from build123d import *

# Parameters (mm, degrees)
BOSS_EXTRUDE1_START = -203.2
BOSS_EXTRUDE1_DEPTH = 203.2
SKETCH15_R          = 5
CUT_EXTRUDE1_DEPTH  = 15


with BuildPart() as part:
    # Sketch12 → Revolve1 (revolve)
    with BuildSketch(Plane.XY, mode=Mode.PRIVATE) as revolve1_sk:
        Polygon((-25.399999994, 0), (-25.399999994, 203.2), (-20.955, 203.2), (-20.955, 165.1), (-19.177, 165.1), (-19.177, 38.1), (-20.955, 38.1), (-20.955, 0), align=None)
    revolve(revolve1_sk.sketch.rotate(Axis((0, 0, 0), (0, 1, 0)), 270), axis=Axis((0, 0, 0), (0, 1, 0)))

    # Sketch13 → Boss-Extrude1 (add)
    with BuildSketch(Plane(origin=(0, 0, 0), x_dir=(-1, 0, 0), z_dir=(0, -1, 0)).offset(BOSS_EXTRUDE1_START)):
        with BuildLine():
            Line((12.584838028, 40.399999994), (-25.399999994, 40.399999994))
            Line((-25.399999994, 40.399999994), (-25.399999994, 0))
            ThreePointArc((-25.399999994, 0), (0, 25.399999994), (25.399999994, 0))
            Line((25.399999994, 0), (25.399999994, 40.399999994))
            Line((25.399999994, 40.399999994), (22.584838028, 40.399999994))
            Line((22.584838028, 40.399999994), (12.584838028, 40.399999994))
        make_face()
    extrude(amount=BOSS_EXTRUDE1_DEPTH)

    # Sketch15 → Cut-Extrude1 (cut)
    with BuildSketch(Plane(origin=(0, 0, -40.399999994), x_dir=(-1, 0, 0), z_dir=(0, 0, -1))):
        with Locations((-12.699999997, 30)):
            Circle(SKETCH15_R)
        with Locations((-12.699999997, 173.2)):
            Circle(SKETCH15_R)
    cut_extrude1 = extrude(amount=-CUT_EXTRUDE1_DEPTH, mode=Mode.SUBTRACT)

    # Mirror1: Cut-Extrude1 across plane
    add(cut_extrude1.mirror(Plane(origin=(0, 0, 0), x_dir=(0, 0, 1), z_dir=(1, 0, 0))), mode=Mode.SUBTRACT)


solid = part.part
Can you work these out from the model? Positions are in its coordinate system, mm. A direction names the side the tool comes from. Coordinates: 2 decimals unless noted, no trailing zeros. Loops run counter-clockwise (first coordinate to the right, second up) from the corner with the lowest first, then second, coordinate; pieces in that order, holes last. Notation, with made-up numbers: (-3, 72.25) - (6, 72.25) arc R29 cw to (6, 103.25) - close; hole circle Ø2 at (-25.5, 46.5). An arc over 180 degrees is marked (long way). Put each result on its own line as item: value. Start each with the question number.
Item 1: Which directions (+Z, -Z, +X, -X, +Y, -Y) give clear straight access to the entire face, cutting with the end or side of a thin tool? Please do faces 1 (the face through (-13, 173, -25.4)), 2 (the face through (0, 203.2, -23)), 3 (the face through (17, 38.1, 9.2)), 4 (the face through (0, 103, -40.4)), 5 (the face through (-17.669, 183.883, -11.265)).
Item 2: If we mould it in two halves opening along Z, with no side actions, what happens to faces 6 (the face through (-17.669, 18.783, -11.265)), 7 (the face through (-19.014, 100.711, 2.496)), 8 (the face through (13, 173, -25.4)), 9 (the face through (13.351, 178.157, -33.005))? For each: +Z half, -Z half, draft (parallel to the pull), parting line (faces both ways), or undercut.
Item 3: If I drill on line 1 along X through (y, z) = (24, 0) (3 decimals); line 2 along Y through (x, z) = (-12.7, -28.25); line 3 along Z through (x, y) = (-10, 51.5), over which ranges is the centre line in solid material (lowest first)?
Item 4: Suppose I cut it at A-A (x = 0). Please give me the cut outline in (y, z) (3 decimals), and give its area (3 significant figures).
Item 5: Suppose I cut it at D-D (z = -8.5). Please give me the cut outline in (x, y), and give its area (3 significant figures).
Item 6: Suppose I cut it at C-C (y = 30). Please give me the cut outline in (x, z) (3 decimals).
Item 7: For pin 1 (9 mm diameter, centred on x = -12.7, y = 173.2, fed in from +Z); pin 2 (5 mm diameter, centred on x = 13.5, y = 173.5, fed in from -Z); pin 3 (10 mm diameter, centred on x = -6.5, z = 9.5, fed in from -Y); pin 4 (5 mm diameter, centred on x = -17, y = 101.5, fed in from +Z), each with a flat end and sliding along its axis, tell me the tip position at first contact or that it passes through.
Item 8: Suppose I cut it at B-B (z = -28.5). Please give me the cut outline in (x, y).
Here are the results:
1. face 1: -Z
1. face 2: +Z, -Z, +X, -X, +Y
1. face 3: -Y
1. face 4: -Z, +X, -X, +Y, -Y
1. face 5: +Y
2. face 6: undercut
2. face 7: undercut
2. face 8: -Z half
2. face 9: draft
3. line 1: -25.4 to -20.955, 20.955 to 25.4
3. line 2: 0 to 25, 35 to 168.2, 178.2 to 203.2
3. line 3: -40.4 to -16.36, 16.36 to 23.35
4. outline: (0, -40.4) - (203.2, -40.4) - (203.2, -20.955) - (165.1, -20.955) - (165.1, -19.177) - (38.1, -19.177) - (38.1, -20.955) - (0, -20.955) - close; (0, 20.955) - (38.1, 20.955) - (38.1, 19.177) - (165.1, 19.177) - (165.1, 20.955) - (203.2, 20.955) - (203.2, 25.4) - (0, 25.4) - close
4. area: 5,310 mm²
5. outline: (-25.4, 0) - (-19.15, 0) - (-19.15, 38.1) - (-17.19, 38.1) - (-17.19, 165.1) - (-19.15, 165.1) - (-19.15, 203.2) - (-25.4, 203.2) - close; (17.19, 38.1) - (19.15, 38.1) - (19.15, 0) - (25.4, 0) - (25.4, 203.2) - (19.15, 203.2) - (19.15, 165.1) - (17.19, 165.1) - close
5. area: 3,040 mm²
6. outline: (-25.4, -40.4) - (-17.7, -40.4) - (-17.7, -25.4) - (-7.7, -25.4) - (-7.7, -40.4) - (7.7, -40.4) - (7.7, -25.4) - (17.7, -25.4) - (17.7, -40.4) - (25.4, -40.4) - (25.4, 0) arc R25.4 ccw to (-25.4, 0) - close; hole circle Ø41.91 at (0, 0)
7. pin 1: z = 24.04
7. pin 2: z = -25.4
7. pin 3: through
7. pin 4: z = 20.85
8. outline: (-25.4, 0) - (25.4, 0) - (25.4, 203.2) - (-25.4, 203.2) - close; hole circle Ø10 at (-12.7, 30); hole circle Ø10 at (-12.7, 173.2); hole circle Ø10 at (12.7, 30); hole circle Ø10 at (12.7, 173.2)
